The drawing under review shows one solid part. Ordinate dimensions are in mm from its lowest x, y, z. A direction names the side the tool comes from. Coordinates: 2 decimals unless noted, no trailing zeros. Order: outer loops, then holes, each group sorted by start corner. A loop starts at its lowest first (then second) coordinate and runs counter-clockwise, first axis right, second up.
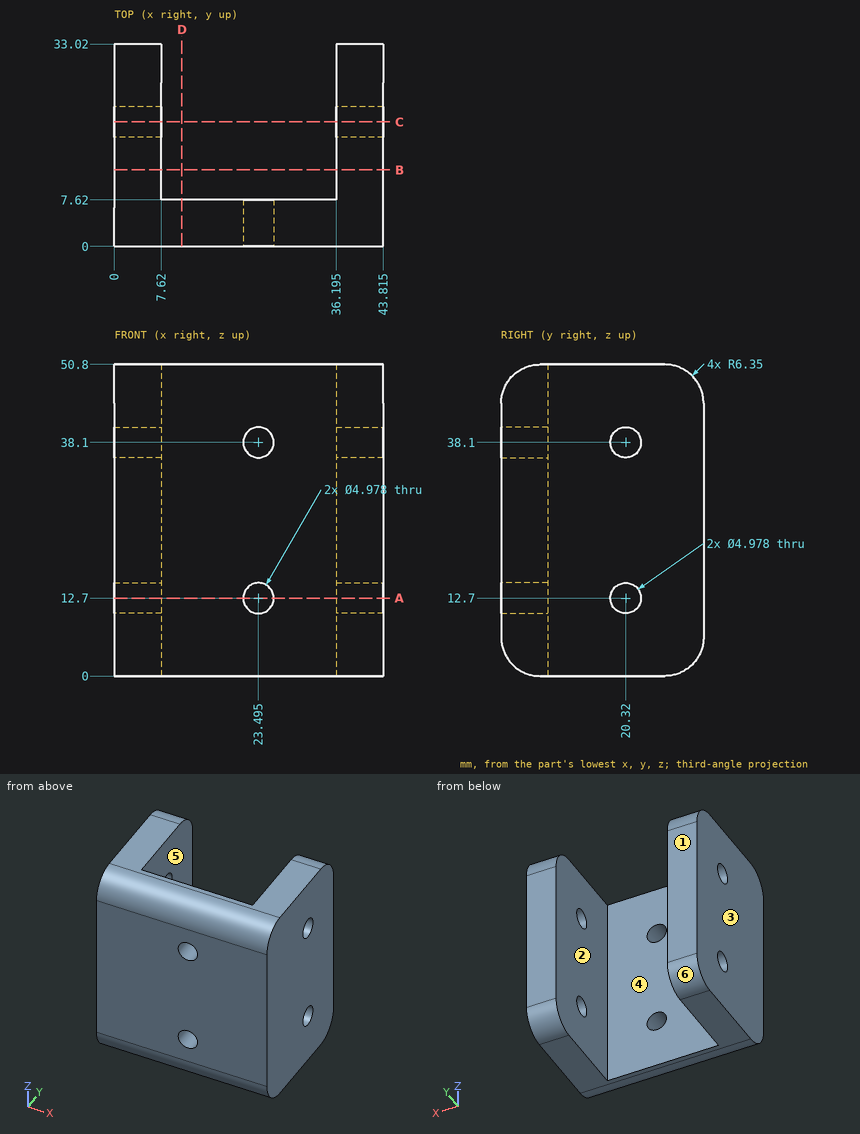
(1) Insertion check: pin 1 Ø12 at (x, z) = (19, 9.5) entering from +Y; pin 2 Ø4 at (x, z) = (23.495, 38.1) entering from -Y. Each pin has a flat end and moves straight along its axis. Give the tip position at first contact, or say it passes through.
(2) Consider section B-B (y = 12.5). Give the boundary of the cut face in (x, z) (1 decimal).
(3) Consider section A-A (z = 12.7). Give the boundary of the cut face in (x, y) (1 decimal).
(4) Consider section D-D (x = 11). Give the boundary of the cut face in (y, z).
(5) The part is to be moulded in two halves that separate along X. For the marked faces 1, 2, 3 and 4, say which applies: +X half, -X half, draft (parallel to the pull), parting line (faces both ways), or undercut.
(6) Wall thickness on line 1 (X direction, y = 16.5, z = 48.5) (1 decimal); line 2 (X direction, y = 4.5, z = 12.7) (1 decimal); line 3 (Y direction, x = 2, z = 38): over which ranges is each line inside the solid? List them lowest first.
(7) Tool access review of the marked faces 5 and 6: name each direction out of +Z, -Z, +X, -X, +Y, -Y from which nothing blocks a thin tool from reaching the whole face with its end or side.
(8) Consider section C-C (y = 20.32). Give the boundary of the cut face in (x, z) (1 decimal).
Findings:
1. pin 1: stops at y = 7.62
1. pin 2: passes through
2. outline: (0, 0) - (7.6, 0) - (7.6, 50.8) - (0, 50.8) - close; (36.2, 0) - (43.8, 0) - (43.8, 50.8) - (36.2, 50.8) - close
3. outline: (0, 0) - (21, 0) - (21, 7.6) - (7.6, 7.6) - (7.6, 17.8) - (0, 17.8) - close; (0, 22.8) - (7.6, 22.8) - (7.6, 33) - (0, 33) - close; (26, 0) - (43.8, 0) - (43.8, 17.8) - (36.2, 17.8) - (36.2, 7.6) - (26, 7.6) - close; (36.2, 22.8) - (43.8, 22.8) - (43.8, 33) - (36.2, 33) - close
4. outline: (0, 6.35) arc R6.35 ccw to (6.35, 0) - (7.62, 0) - (7.62, 50.8) - (6.35, 50.8) arc R6.35 ccw to (0, 44.45) - close
5. face 1: draft
5. face 2: undercut
5. face 3: -X half
5. face 4: undercut
6. line 1: x = 0 to 7.6, 36.2 to 43.8
6. line 2: x = 0 to 21, 26 to 43.8
6. line 3: y = 0 to 17.83, 22.81 to 33.02
7. face 5: +Z, -Z, +Y
7. face 6: -Z, +X, -X, +Y
8. outline: (0, 0) - (7.6, 0) - (7.6, 10.2) - (0, 10.2) - close; (0, 15.2) - (7.6, 15.2) - (7.6, 35.6) - (0, 35.6) - close; (0, 40.6) - (7.6, 40.6) - (7.6, 50.8) - (0, 50.8) - close; (36.2, 0) - (43.8, 0) - (43.8, 10.2) - (36.2, 10.2) - close; (36.2, 15.2) - (43.8, 15.2) - (43.8, 35.6) - (36.2, 35.6) - close; (36.2, 40.6) - (43.8, 40.6) - (43.8, 50.8) - (36.2, 50.8) - close
